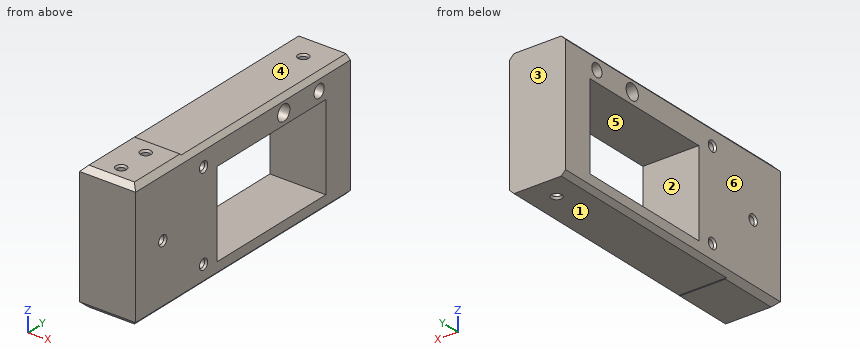
Solid Edge part; units mm, degrees
sketch "Sketch1" plane through (0, 0, 0) normal (0, 0, 1) x (1, 0, 0)
  line L0 (-16, -30) -> (16, -30)
  line L1 (16, -30) -> (16, 30)
  line L2 (16, 30) -> (-16, 30)
  line L3 (-16, 30) -> (-16, -30)
  dimension "D1" = 16
  dimension "D2" = 16
extrude "Protrusion1" add sketch "Sketch1" along normal blind 73
sketch "Sketch2" plane through (0, 0, 73) normal (0, 0, 1) x (1, 0, 0)
  circle A0 centre (0, -20) radius 2.35
  circle A1 centre (0, -2) radius 2.35
extrude "Extrusionsausschnitt_1" cut sketch "Sketch2" against normal blind 36
chamfer "Fase_3" distance 0.7 angle 60 2 edges at (-2.35, -2, 73) (-2.35, -20, 73) measured on face at (-10.9867, -19.4, 73)
chamfer "Fase_6" distance 3 angle 45 4 edges at (-16, 0, 73) (-16, 0, 0) (16, 0, 73) (16, 0, 0)
chamfer "Fase_7" distance 3 angle 45 2 edges at (0, -30, 73) (0, -30, 0)
sketch "Sketch3" plane through (-16, 0, 36.5) normal (-1, 0, 0) x (0, -1, 0)
  circle A0 centre (-20, 25) radius 2.35
  circle A1 centre (-20, -25) radius 2.35
  circle A2 centre (10, 0) radius 2.35
  dimension "D1" = 20
extrude "Cutout1" cut sketch "Sketch3" against normal through all
chamfer "Fase_9" distance 0.7 angle 60 6 edges at (-16, 22.35, 61.5) (-16, -7.65, 36.5) (-16, 22.35, 11.5) (16, 20, 59.15) (16, 20, 9.15) (16, -10, 34.15) measured on face at (-16, 20.6, 58.1633) measured on face at (16, -20.6, 58.1633)
sketch "Sketch4" plane through (-16, 0, 36.5) normal (-1, 0, 0) x (0, -1, 0)
  line L0 (-6.5, 36.5) -> (-30, 36.5)
  line L1 (-30, 36.5) -> (-30, 36)
  line L2 (-30, 36) -> (-6.5, 36)
  line L3 (-6.5, 36) -> (-6.5, 36.5)
  line L4 (-30, -36.5) -> (-6.5, -36.5)
  line L5 (-6.5, -36.5) -> (-6.5, -36)
  line L6 (-6.5, -36) -> (-30, -36)
  line L7 (-30, -36) -> (-30, -36.5)
  dimension "D1" = 30
  dimension "D2" = 30
extrude "Cutout2" cut sketch "Sketch4" against normal through all
sketch "Sketch5" plane through (0, 30, 36.5) normal (0, 1, 0) x (1, 0, 0)
  line L0 (-16, 33.5) -> (-13.5, 36)
  line L1 (-13.5, 36) -> (13.5, 36)
  line L2 (13.5, 36) -> (16, 33.5)
  line L3 (16, 33.5) -> (16, -33.5)
  line L4 (16, -33.5) -> (13.5, -36)
  line L5 (13.5, -36) -> (-13.5, -36)
  line L6 (-13.5, -36) -> (-16, -33.5)
  line L7 (-16, -33.5) -> (-16, 33.5)
extrude "Extrusionsausprägung_2" add sketch "Sketch5" along normal blind 26
sketch "Sketch6" plane through (0, 56, 36.5) normal (0, 1, 0) x (-1, 0, 0)
  line L0 (-13.5, 36) -> (-16, 33.5)
  line L1 (-16, 33.5) -> (-16, -33.5)
  line L2 (-16, -33.5) -> (-13.5, -36)
  line L3 (-13.5, -36) -> (13.5, -36)
  line L4 (13.5, -36) -> (16, -33.5)
  line L5 (16, -33.5) -> (16, 33.5)
  line L6 (16, 33.5) -> (13.5, 36)
  line L7 (13.5, 36) -> (-13.5, 36)
extrude "Extrusionsausprägung_3" add sketch "Sketch6" along normal blind 72
sketch "Sketch7" plane through (16, 47, 36.5) normal (1, 0, 0) x (0, 1, 0)
  line L0 (-17, 21) -> (63, 21)
  line L1 (63, 21) -> (63, -28)
  line L2 (63, -28) -> (-17, -28)
  line L3 (-17, -28) -> (-17, 21)
  dimension "D1" = 17
extrude "Cutout3" cut sketch "Sketch7" against normal through all
sketch "Sketch8" plane through (0, 65.25, 72.5) normal (0, 0, 1) x (0, 1, 0)
  circle A0 centre (48.75, 0) radius 2.35
  dimension "D1" = 48.75
extrude "Cutout4" cut sketch "Sketch8" against normal through all
chamfer "Fase_11" distance 0.7 angle 60 2 edges at (-2.35, 114, 0.5) (0, 111.65, 72.5) measured on face at (8.73, 108.965, 72.5) measured on face at (8.73, 25.535, 0.5)
sketch "Sketch9" plane through (-16, 49, 36.5) normal (-1, 0, 0) x (0, -1, 0)
  circle A0 centre (-56, 27.5) radius 3.75
extrude "Cutout5" cut sketch "Sketch9" against normal through all
sketch "Sketch10" plane through (-16, 49, 36.5) normal (-1, 0, 0) x (0, -1, 0)
  circle A0 centre (-30, 27.5) radius 4.5
extrude "Cutout6" cut sketch "Sketch10" against normal through all
properties material "Nylon, allgemein"
Geometry: final body of the model. Coordinates: model frame, mm. Face numbers are marked on the shaded views. A direction names the side the tool comes from. Give positions to 0.01 mm unless a question says otherwise; leave off trailing zeros. Loops run counter-clockwise (first coordinate to the right, second up) from the corner with the lowest first, then second, coordinate; pieces in that order, holes last. Notation, with made-up numbers: (15, 36.25) - (51, 36.25) arc R12 ccw to (51, 48.25) - close; hole circle Ø3 at (-40, 84.5). An arc over 180 degrees is marked (long way). One line per question, with ' | ' between items. Start each with the question number.
(1) Section query D-D on x = 5. Return loops of the section in (y, z).
(2) Section query A-A on z = 19.5. Return loops of the section in (x, y), then the cut area to 3 significant figures.
(3) Reachability of the marked faces 1, 2 and 3 from +Z, -Z, +X, -X, +Y, -Y: full face, straight path, thin tool, end or side. Return the list, or none.
(4) Section query C-C on y = 20. Return loops of the section in (x, z).
(5) Contact query for flat-ended pins moving along their axis: pin 1 (1.5 mm diameter, centred on x = 10.5, y = 99.5, fed in from -Z); pin 2 (5.5 mm diameter, centred on y = -10, z = 36.5, fed in from -X); pin 3 (6 mm diameter, centred on y = 20, z = 11.5, fed in from +X). Output: stop coordinate, or through.
(6) Section query B-B on y = 88. Return loops of the section in (x, z), then the cut area to 4 significant figures.
(7) Ray query, line 1 (Y direction, x = 0, z = 49.5); line 2 (Z direction, x = 9, y = 20); line 3 (Y direction, x = -14.5, z = 64.5). Return the intervals inside material, ascending. Write a range as from..to.
(8) Pull-direction query (Z, two-part tool) for the marked faces 4, 5 and 6; classes: released by +Z, released by -Z, zero draft, split by the parting line, or undercut.
The answers:
1) outline: (-30, 3) - (-27, 0) - (6.5, 0) - (6.5, 0.5) - (128, 0.5) - (128, 72.5) - (6.5, 72.5) - (6.5, 73) - (-27, 73) - (-30, 70) - close; hole circle Ø4.7 at (-10, 36.5); hole circle Ø4.7 at (20, 11.5); hole circle Ø4.7 at (20, 61.5); hole (30, 8.5) - (110, 8.5) - (110, 57.5) - (30, 57.5) - close; hole circle Ø9 at (79, 64); hole circle Ø7.5 at (105, 64)
2) outline: (-16, -30) - (16, -30) - (16, 30) - (-16, 30) - close; (-16, 110) - (16, 110) - (16, 128) - (-16, 128) - close; hole circle Ø4.7 at (0, 114) | area: 2,480 mm2
3) face 1: -Z, +X, -X, +Y | face 2: +X, -X | face 3: +Z, -Z, +X, -X, +Y
4) outline: (-16, 3) - (-13.5, 0.5) - (13.5, 0.5) - (16, 3) - (16, 8.45) - (14.79, 9.15) - (-14.79, 9.15) - (-16, 8.45) - close; (-16, 14.55) - (-14.79, 13.85) - (14.79, 13.85) - (16, 14.55) - (16, 58.45) - (14.79, 59.15) - (-14.79, 59.15) - (-16, 58.45) - close; (-16, 64.55) - (-14.79, 63.85) - (14.79, 63.85) - (16, 64.55) - (16, 70) - (13.5, 72.5) - (-13.5, 72.5) - (-16, 70) - close
5) pin 1: z = 0.5 | pin 2: x = -15.48 | pin 3: x = 15.91
6) outline: (-16, 3) - (-13.5, 0.5) - (13.5, 0.5) - (16, 3) - (16, 8.5) - (-16, 8.5) - close; (-16, 57.5) - (16, 57.5) - (16, 70) - (13.5, 72.5) - (-13.5, 72.5) - (-16, 70) - close | area: 723.5 mm2
7) line 1: -30..-22.35, -17.65..-4.35, 0.35..30, 110..111.65, 116.35..128 | line 2: 0.5..9.15, 13.85..59.15, 63.85..72.5 | line 3: -30..74.53, 83.47..101.28, 108.72..128
8) face 4: released by +Z | face 5: undercut | face 6: zero draft
